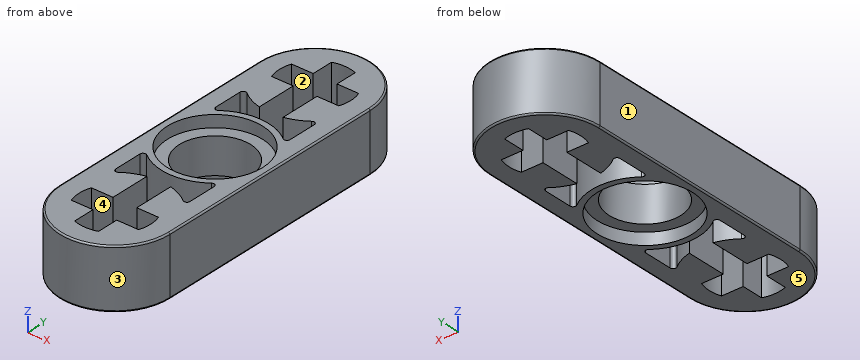
```python
from build123d import *

# Parameters (mm, degrees)
BOSS_EXTRUDE1_DEPTH = 4
CUT_EXTRUDE1_DEPTH  = 21.439667316
CUT_EXTRUDE2_DEPTH  = 21.439667316
FILLET1_R           = 0.1


with BuildPart() as part:
    # Sketch1 → Boss-Extrude1 (new body)
    with BuildSketch(Plane(origin=(0, 0, -2), x_dir=(-1, 0, 0), z_dir=(0, 0, -1))):
        with BuildLine():
            Line((-3.7, 0), (-3.7, -16))
            ThreePointArc((-3.7, -16), (0, -19.7), (3.7, -16))
            Line((3.7, -16), (3.7, 0))
            ThreePointArc((3.7, 0), (0, 3.7), (-3.7, 0))
        make_face()
    extrude(amount=-BOSS_EXTRUDE1_DEPTH)

    # Sketch2 → Cut-Extrude1 (cut, through all)
    with BuildSketch(Plane(origin=(0, 0, -2), x_dir=(-1, 0, 0), z_dir=(0, 0, -1))):
        with BuildLine():
            Line((-0.8, -0.8), (-0.8, -3.509985755))
            ThreePointArc((-0.8, -3.509985755), (-1.523912922, -3.261547088), (-2.178947368, -2.865691603))
            ThreePointArc((-2.178947368, -2.865691603), (-2.388852332, -2.845717276), (-2.5, -3.024896692))
            Line((-2.5, -3.024896692), (-2.5, -4.975103308))
            ThreePointArc((-2.5, -4.975103308), (-2.388852332, -5.154282724), (-2.178947368, -5.134308397))
            ThreePointArc((-2.178947368, -5.134308397), (0, -4.4), (2.178947368, -5.134308397))
            ThreePointArc((2.178947368, -5.134308397), (2.388852332, -5.154282724), (2.5, -4.975103308))
            Line((2.5, -4.975103308), (2.5, -3.024896692))
            ThreePointArc((2.5, -3.024896692), (2.388852332, -2.845717276), (2.178947368, -2.865691603))
            ThreePointArc((2.178947368, -2.865691603), (1.523912922, -3.261547088), (0.8, -3.509985755))
            Line((0.8, -3.509985755), (0.8, -0.8))
            Line((0.8, -0.8), (2.2627417, -0.8))
            ThreePointArc((2.2627417, -0.8), (2.4, 0), (2.2627417, 0.8))
            Line((2.2627417, 0.8), (0.8, 0.8))
            Line((0.8, 0.8), (0.8, 2.2627417))
            ThreePointArc((0.8, 2.2627417), (0, 2.4), (-0.8, 2.2627417))
            Line((-0.8, 2.2627417), (-0.8, 0.8))
            Line((-0.8, 0.8), (-2.2627417, 0.8))
            ThreePointArc((-2.2627417, 0.8), (-2.4, 0), (-2.2627417, -0.8))
            Line((-2.2627417, -0.8), (-0.8, -0.8))
        make_face()
    extrude(amount=-CUT_EXTRUDE1_DEPTH, mode=Mode.SUBTRACT)

    # Sketch3 → Cut-Extrude2 (cut, through all)
    with BuildSketch(Plane.XY.offset(2)):
        with BuildLine():
            Line((2.5, -12.975103308), (2.5, -11.024896692))
            ThreePointArc((2.5, -11.024896692), (2.388852332, -10.845717276), (2.178947368, -10.865691603))
            ThreePointArc((2.178947368, -10.865691603), (0, -11.6), (-2.178947368, -10.865691603))
            ThreePointArc((-2.178947368, -10.865691603), (-2.388852332, -10.845717276), (-2.5, -11.024896692))
            Line((-2.5, -11.024896692), (-2.5, -12.975103308))
            ThreePointArc((-2.5, -12.975103308), (-2.388852332, -13.154282724), (-2.178947368, -13.134308397))
            ThreePointArc((-2.178947368, -13.134308397), (-1.523912922, -12.738452912), (-0.8, -12.490014245))
            Line((-0.8, -12.490014245), (-0.8, -15.2))
            Line((-0.8, -15.2), (-2.2627417, -15.2))
            ThreePointArc((-2.2627417, -15.2), (-2.4, -16), (-2.2627417, -16.8))
            Line((-2.2627417, -16.8), (-0.8, -16.8))
            Line((-0.8, -16.8), (-0.8, -18.2627417))
            ThreePointArc((-0.8, -18.2627417), (0, -18.4), (0.8, -18.2627417))
            Line((0.8, -18.2627417), (0.8, -16.8))
            Line((0.8, -16.8), (2.2627417, -16.8))
            ThreePointArc((2.2627417, -16.8), (2.4, -16), (2.2627417, -15.2))
            Line((2.2627417, -15.2), (0.8, -15.2))
            Line((0.8, -15.2), (0.8, -12.490014245))
            ThreePointArc((0.8, -12.490014245), (1.523912922, -12.738452912), (2.178947368, -13.134308397))
            ThreePointArc((2.178947368, -13.134308397), (2.388852332, -13.154282724), (2.5, -12.975103308))
        make_face()
    extrude(amount=-CUT_EXTRUDE2_DEPTH, mode=Mode.SUBTRACT)

    # Sketch4 → Cut-Revolve1 (revolve, cut)
    with BuildSketch(Plane(origin=(0, -8, 0), x_dir=(1, 0, 0), z_dir=(0, 1, 0))):
        Polygon((3.2, 2), (0, 2), (0, -2), (3.2, -2), (3.2, -1.2), (2.4, -1.2), (2.4, 1.2), (3.2, 1.2), align=None)
    revolve(axis=Axis((0, -8, -2), (0, 0, 1)), mode=Mode.SUBTRACT)

    # Fillet1
    fillet1_edges = [part.edges().sort_by_distance(p)[0] for p in [
        (0, -19.7, 2),
        (-3.7, -8, 2),
        (0, 3.7, 2),
        (-3.7, -8, -2),
        (0, -19.7, -2),
        (3.7, -8, -2),
        (0, 3.7, -2),
        (3.7, -8, 2),
    ]]
    fillet(fillet1_edges, radius=FILLET1_R)


solid = part.part
```
Geometry: final body of the model. Coordinates: model frame, mm. Face numbers are marked on the shaded views. A direction names the side the tool comes from. Round coordinates to 2 decimals unless told otherwise and drop trailing zeros. Write each loop counter-clockwise with the first axis right and the second up, starting at its lowest first coordinate (ties: lowest second). Pieces come first, ordered by that corner, then holes. Notation, with made-up numbers: M -32.75,57.25 L 17.25,57.25 A27 ccw 17.25,80.25 Z; hole C 58.25,27 d7. An arc over 180 degrees is marked long. Answer in a Markdown table with one row per item. Add a question column.
(1) Ray query, L1, parallel to Y at x = 0, z = 0.35; L2, parallel to Y at x = 0, z = -1.75; L3, parallel to X at y = -4.25, z = 0.4. Return the intervals inside material, ascending.
(2) Cut plane A-A, the plane y = -1. Return the cut outline in (x, z).
(3) Cut plane D-D, the plane z = 1.4. Give the number of separate pieces and of enclosed holes in the cut face, then the cut area to 3 significant figures.
(4) Cut plane C-C, the plane y = -3.75. Return the cut outline in (x, z), then the cut area to 3 significant figures.
(5) Cut plane B-B, the plane x = 0. Return the cut outline in (y, z), then the cut area to 3 significant figures.
(6) Reachability of the marked faces 4 and 5 from +Z, -Z, +X, -X, +Y, -Y: full face, straight path, thin tool, end or side. Return the list, or none.
(7) Contact query for flat-ended pins moving along their axis: pin 1 (1.6 mm diameter, centred on x = -2, z = -1, fed in from +Y); pin 2 (1.2 mm diameter, centred on x = 1.5, z = 0, fed in from -Y); pin 3 (1.2 mm diameter, centred on y = -17.5, z = 1, fed in from -X); pin 4 (4 mm diameter, centred on x = 1, y = -9.5, fed in from +Z). Output: stop coordinate, or through.
(8) Draft query along Y for the marked faces 1, 2 and 3. Return one class per face: pulls with the +Y half, pulls with the -Y half, needs draft (parallel to the pull), parting line crosses it, or undercut.
Established:
| question | item | result |
|---|---|---|
| 1 | L1 | -19.7 to -18.4, -11.6 to -10.4, -5.6 to -4.4, 2.4 to 3.7 |
| 1 | L2 | -19.7 to -18.4, -11.6 to -11.2, -4.8 to -4.4, 2.4 to 3.7 |
| 1 | L3 | -3.7 to -2.5, 2.5 to 3.7 |
| 2 | outline | M -3.7,-1.9 A0.1 ccw -3.6,-2 L -0.8,-2 L -0.8,2 L -3.6,2 A0.1 ccw -3.7,1.9 Z; M 0.8,-2 L 3.6,-2 A0.1 ccw 3.7,-1.9 L 3.7,1.9 A0.1 ccw 3.6,2 L 0.8,2 Z |
| 3 | separate pieces | 1 |
| 3 | enclosed holes | 3 |
| 3 | area | 86.3 mm² |
| 4 | outline | M -3.7,-1.9 A0.1 ccw -3.6,-2 L -2.5,-2 L -2.5,2 L -3.6,2 A0.1 ccw -3.7,1.9 Z; M 2.5,-2 L 3.6,-2 A0.1 ccw 3.7,-1.9 L 3.7,1.9 A0.1 ccw 3.6,2 L 2.5,2 Z |
| 4 | area | 9.59 mm² |
| 5 | outline | M -19.7,-1.9 A0.1 ccw -19.6,-2 L -18.4,-2 L -18.4,2 L -19.6,2 A0.1 ccw -19.7,1.9 Z; M -11.6,-2 L -11.2,-2 L -11.2,-1.2 L -10.4,-1.2 L -10.4,1.2 L -11.2,1.2 L -11.2,2 L -11.6,2 Z; M -5.6,-1.2 L -4.8,-1.2 L -4.8,-2 L -4.4,-2 L -4.4,2 L -4.8,2 L -4.8,1.2 L -5.6,1.2 Z; M 2.4,-2 L 3.6,-2 A0.1 ccw 3.7,-1.9 L 3.7,1.9 A0.1 ccw 3.6,2 L 2.4,2 Z |
| 5 | area | 17.4 mm² |
| 6 | face 4 | +Z, -Z |
| 6 | face 5 | -Z, +X, -X, +Y, -Y |
| 7 | pin 1 | y = 3.5 |
| 7 | pin 2 | y = -19.59 |
| 7 | pin 3 | x = -3.59 |
| 7 | pin 4 | z = 2 |
| 8 | face 1 | needs draft |
| 8 | face 2 | undercut |
| 8 | face 3 | pulls with the -Y half |
